Part model, mm, in its own coordinate system. A direction names the side the tool comes from. Coordinates: 2 decimals unless noted, no trailing zeros. Loops run counter-clockwise (first coordinate to the right, second up) from the corner with the lowest first, then second, coordinate; pieces in that order, holes last. Notation, with made-up numbers: M 13.25,17.5 L 65.25,17.5 A17 ccw 65.25,27.5 Z; hole C -15.5,79 d1. An arc over 180 degrees is marked long. Use CSV: the item, a comma, the result in double quotes. Start each with the question number.
from build123d import *

# Parameters (mm, degrees)
ESQUISSE2_R                  = 16
ESQUISSE2_R_2                = 14
EXTRUSION5_DEPTH             = 213
ENL_V_MAT_EXTRU_1_DEPTH      = 17
ENL_V_MAT_EXTRU_1_DEPTH_BACK = 17
ENL_V_MAT_EXTRU_2_DEPTH      = 68.17581801


with BuildPart() as part:
    # Esquisse2 → Extrusion5 (new body)
    with BuildSketch(Plane(origin=(148.407000681, 477.467655605, 0), x_dir=(-0.954935311, 0.296814001, 0), z_dir=(0.296814001, 0.954935311, 0))):
        Circle(ESQUISSE2_R)
        Circle(ESQUISSE2_R_2, mode=Mode.SUBTRACT)
    extrude(amount=-EXTRUSION5_DEPTH)

    # Esquisse12 → Enlèv. mat.-Extru.1 (cut, two sides)
    with BuildSketch(Plane.XY) as enl_v_mat_extru_1_sk:
        with BuildLine():
            Line((67.680548401, 271.653443505), (76.584968442, 300.301502841))
            ThreePointArc((76.584968442, 300.301502841), (81.480701144, 306.1845671), (89.102461568, 306.88271594))
            Line((89.102461568, 306.88271594), (117.750520904, 297.978295899))
            ThreePointArc((117.750520904, 297.978295899), (132.458181552, 285.738964145), (134.20355365, 266.684563085))
            Line((134.20355365, 266.684563085), (125.29913361, 238.036503748))
            ThreePointArc((125.29913361, 238.036503748), (120.403400908, 232.153439489), (112.781640484, 231.45529065))
            Line((112.781640484, 231.45529065), (84.133581147, 240.359710691))
            ThreePointArc((84.133581147, 240.359710691), (69.4259205, 252.599042445), (67.680548401, 271.653443505))
        make_face()
    extrude(amount=ENL_V_MAT_EXTRU_1_DEPTH, mode=Mode.SUBTRACT)
    extrude(enl_v_mat_extru_1_sk.sketch, amount=-ENL_V_MAT_EXTRU_1_DEPTH_BACK, mode=Mode.SUBTRACT)

    # Esquisse13 → Enlèv. mat.-Extru.2 (cut, through all)
    with BuildSketch(Plane(origin=(0, 0, 0), x_dir=(0, 0, -1), z_dir=(0.954935311, -0.296814001, 0))):
        with BuildLine():
            Line((-1.75, 500), (1.75, 500))
            Line((1.75, 500), (1.75, 473.75))
            ThreePointArc((1.75, 473.75), (0, 472), (-1.75, 473.75))
            Line((-1.75, 473.75), (-1.75, 500))
        make_face()
    extrude(amount=ENL_V_MAT_EXTRU_2_DEPTH, mode=Mode.SUBTRACT)


solid = part.part
1. Slice it at A-A, the plane z = 8.5. List the corners of the cut face in (x, y), and give its area (3 significant figures).
2. Tool access for faces 1 (the face through (159, 460, 1.75)), 2 (the face through (79.986, 305.22, 0.069)): list every direction of +Z, -Z, +X, -X, +Y, -Y with a clear straight run to the whole face (end or side of a thin tool).
3. Pin check, flat tips, straight feed: pin 1 (12 mm diameter, centred on x = 99, z = 10, fed in from -Y); pin 2 (4 mm diameter, centred on y = 330, z = 9.5, fed in from +X); pin 3 (10 mm diameter, centred on y = 355, z = -1.5, fed in from -X). Stop position of each tip, or through.
4. Slice it at B-B, the plane z = -6. List the corners of the cut face in (x, y), and give its area (3 significant figures).
5. Two-plate mould, pull along Z, no slides. Class faces 3 (the face through (139.405, 480.266, 10.741)), 4 (the face through (109.06, 394.45, -5.36)), 5 (the face through (106.42, 392.17, -6.13)): pulls with the +Z half, pulls with the -Z half, needs draft (parallel to the pull), parting line crosses it, or undercut.
6. Wall check: probe 1 along X at (y, z) = (347, -12); probe 2 along X at (y, z) = (470, -5); probe 3 along Z at (x, y) = (136, 457.5). Give the ranges that are in metal, low to high.
Found:
1,outline,"M 80.86,305.83 A10 cw 83.79,307.05 L 137.78,480.77 L 135.46,481.49 Z; M 105.46,301.8 L 107.78,301.08 L 161.35,473.44 L 159.03,474.17 Z"
1,area,"883 mm^2"
2,face 1,"+X, +Y"
2,face 2,"+Z, -Z, -Y"
3,pin 1,"y = 301.94"
3,pin 2,"x = 117.53"
3,pin 3,"x = 92.07"
4,outline,"M 79.09,304.43 A10 cw 82,306.44 L 136.33,481.22 L 134.24,481.87 Z; M 106.91,301.35 L 109,300.7 L 162.57,473.07 L 160.49,473.71 Z"
4,area,"796 mm^2"
5,face 3,"needs draft"
5,face 4,"undercut"
5,face 5,"parting line crosses it"
6,probe 1,"96.77 to 100.3, 115.41 to 118.94"
6,probe 2,"130.17 to 132.39, 159.78 to 162"
6,probe 3,"-14.86 to -12.69, 12.69 to 14.86"
